from build123d import *

# Parameters (mm, degrees)
BOSS_EXTRUDE1_DEPTH = 32
SKETCH2_W           = 3.5
SKETCH2_H           = 15
CUT_EXTRUDE1_DEPTH  = 86.609578903


with BuildPart() as part:
    # Sketch1 → Boss-Extrude1 (new, symmetric)
    with BuildSketch(Plane(origin=(0, 0, 0), x_dir=(0, 0, -1), z_dir=(1, 0, 0))):
        Polygon((0, 0), (-4, 0), (-4, 30), (-30, 49.1), (-47, 42.9), (-47, 46.9), (0, 64), align=None)
    extrude(amount=BOSS_EXTRUDE1_DEPTH, both=True)

    # Sketch2 → Cut-Extrude1 (cut, through all)
    with BuildSketch(Plane(origin=(0, 0, 0), x_dir=(-1, 0, 0), z_dir=(0, 0, -1))):
        with Locations((20, 15)):
            Rectangle(SKETCH2_W, SKETCH2_H)
        with Locations((-20, 15)):
            Rectangle(SKETCH2_W, SKETCH2_H)
    extrude(amount=-CUT_EXTRUDE1_DEPTH, mode=Mode.SUBTRACT)


solid = part.part
Check sheet for the modelled part. Datum: model origin and axes. Units: mm. A direction names the side the tool comes from. Coordinates: 2 decimals unless noted, no trailing zeros. Write each loop counter-clockwise with the first axis right and the second up, starting at its lowest first coordinate (ties: lowest second). Pieces come first, ordered by that corner, then holes.
Item 1: Access from +Z, -Z, +X, -X, +Y, -Y to the whole of each face (thin tool, end or side, straight path). Record for faces 4 (the face through (0, 15, 4)), 5 (the face through (-32, 44, 13)), 6 (the face through (0.45, 55.33, 23.83)), 7 (the face through (-20, 22.5, 2)), 8 (the face through (0.448, 46.043, 38.381)).
Numbers:
face 4: +Z, +X, -X, -Y
face 5: +Z, -Z, -X, +Y, -Y
face 6: +Z, +X, -X, +Y
face 7: +Z, -Z
face 8: +X, -X, -Y
Item 2: Depth check by flat-ended pin: pin 1 Ø3 at (x, z) = (-20, 2.5) entering from +Y; pin 2 Ø2 at (x, z) = (25, 14.5) entering from +Y; pin 3 Ø24 at (x, y) = (-6.5, 19.5) entering from +Z. Enter the tip coordinate at first touch or a pass-through.
Numbers:
pin 1: stops at y = 63.64
pin 2: stops at y = 59.09
pin 3: stops at z = 6.04
Item 3: Scan lines: probe 1 along Z at (x, y) = (28, 21); probe 2 along Z at (x, y) = (-22, 36.5); probe 3 along Y at (x, z) = (-15.5, 30.5). Record each from-to range of solid material in increasing order.
Numbers:
probe 1: z = 0 to 4
probe 2: z = 0 to 12.85
probe 3: y = 48.92 to 52.9
Item 4: Cross-section at B-B on y = 46. Record the boundary of the cut face in (x, z).
Numbers:
outline: (-32, 0) - (32, 0) - (32, 25.78) - (-32, 25.78) - close; (-32, 38.5) - (32, 38.5) - (32, 47) - (-32, 47) - close
Item 5: Cross-section at A-A on x = -20. Record the boundary of the cut face in (y, z), then the cut area to 3 significant figures.
Numbers:
outline: (0, 0) - (7.5, 0) - (7.5, 4) - (0, 4) - close; (22.5, 0) - (64, 0) - (46.9, 47) - (42.9, 47) - (49.1, 30) - (30, 4) - (22.5, 4) - close
area: 736 mm2
Item 6: Mould release check, pull along Y, two halves, no side actions. Record for faces 1 (the face through (21.75, 15, 2)), 2 (the face through (0, 0, 2)), 3 (the face through (32, 44, 13)): released by +Y, released by -Y, zero draft, split by the parting line, or undercut.
Numbers:
face 1: undercut
face 2: released by -Y
face 3: zero draft
Item 7: Cross-section at D-D on z = 11. Record the boundary of the cut face in (x, y), then the cut area to 3 significant figures.
Numbers:
outline: (-32, 35.14) - (32, 35.14) - (32, 60) - (-32, 60) - close
area: 1,590 mm2
Item 8: Cross-section at C-C on y = 13. Record the boundary of the cut face in (x, z).
Numbers:
outline: (-32, 0) - (-21.75, 0) - (-21.75, 4) - (-32, 4) - close; (-18.25, 0) - (18.25, 0) - (18.25, 4) - (-18.25, 4) - close; (21.75, 0) - (32, 0) - (32, 4) - (21.75, 4) - close
